Input: part model. Units: mm. Frame: model coordinates. Face numbers are marked on the shaded views. A direction names the side the tool comes from. Coordinates: 2 decimals unless noted, no trailing zeros. Write each loop counter-clockwise with the first axis right and the second up, starting at its lowest first coordinate (ties: lowest second). Pieces come first, ordered by that corner, then holes. Notation, with made-up numbers: M 41,30.25 L 59,30.25 A32 cw 59,60.25 Z; hole C 61.5,-37 d4. An arc over 180 degrees is marked long. Use one line per item in the form item = value.
from build123d import *

# Parameters (mm, degrees)
RECPAT_COUNT       = 2
RECPAT_ANGLE       = 90
BOSS_EXTRU_1_START = 10
ESQUISSE1_R        = 2
BOSS_EXTRU_1_DEPTH = 10


with BuildPart() as part:
    # Fillet1: read off the stored shape, not the designer's step
    # Fillet1 outline → Fillet1 (revolve)
    with BuildSketch(Plane.YX):
        with BuildLine():
            Line((2, 3.3), (2, 8.1))
            Line((2, 8.1), (0, 8.1))
            Line((0, 8.1), (0, 0))
            ThreePointArc((0, 0), (2.027933458, 0.324444488), (3.853420198, 1.265388956))
            ThreePointArc((3.853420198, 1.265388956), (3.961271902, 1.392873227), (4, 1.555305874))
            Line((4, 1.555305874), (4, 3.1))
            Line((4, 3.1), (2.2, 3.1))
            ThreePointArc((2.2, 3.1), (2.058578644, 3.158578644), (2, 3.3))
        make_face()
    revolve(axis=Axis((0, 0, 0), (1, 0, 0)))

    # Sketch3 → Recess section 0
    with BuildSketch(Plane(origin=(0, 0, 0), x_dir=(0, 0, -1), z_dir=(1, 0, 0))):
        with BuildLine():
            Line((0.515, -2.15), (-0.515, -2.15))
            Line((-0.515, -2.15), (-0.515, 2.15))
            Line((-0.515, 2.15), (0.515, 2.15))
            Line((0.515, 2.15), (0.515, -2.15))
        make_face()
    # Sketch4 → Recess section 1
    with BuildSketch(Plane(origin=(2.34, 0, 0), x_dir=(0, 0, -1), z_dir=(1, 0, 0))):
        with BuildLine():
            Line((0.515, -0.983319232), (-0.515, -0.983319232))
            Line((-0.515, -0.983319232), (-0.515, 0.983319232))
            Line((-0.515, 0.983319232), (0.515, 0.983319232))
            Line((0.515, 0.983319232), (0.515, -0.983319232))
        make_face()
    recess = loft(mode=Mode.SUBTRACT)

    # RecPat: Recess ×2 about axis
    recpat_axis = Axis((0, 0, 0), (1, 0, 0))
    for i in range(1, RECPAT_COUNT):
        add(recess.rotate(recpat_axis, i * RECPAT_ANGLE / (RECPAT_COUNT - 1)), mode=Mode.SUBTRACT)

    # RecCorSke → RecessCore (revolve, cut)
    with BuildSketch(Plane.XY, mode=Mode.PRIVATE) as recesscore_sk:
        Polygon((0, 0), (0, 1.01462874), (2.34, 0.851), (2.616506661, 0), align=None)
    revolve(recesscore_sk.sketch.rotate(Axis((-3.175, 0, 0), (1, 0, 0)), 90), axis=Axis((-3.175, 0, 0), (1, 0, 0)), mode=Mode.SUBTRACT)

    # Esquisse1 → Boss.-Extru.1 (add)
    with BuildSketch(Plane(origin=(8.1, 0, 0), x_dir=(0, 0, -1), z_dir=(1, 0, 0)).offset(BOSS_EXTRU_1_START)):
        with Locations(Location((0, 0, 0), (0, 0, 180))):
            Circle(ESQUISSE1_R)
    extrude(amount=-BOSS_EXTRU_1_DEPTH)


solid = part.part
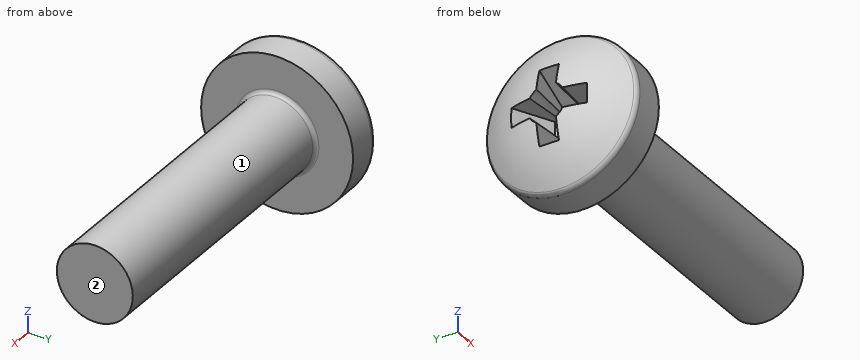
(1) Set-up query: the marked faces 1 and 2. Return all of +Z, -Z, +X, -X, +Y, -Y with unobstructed straight access to the full face (end or side cutting, diameter ignored); none if empty.
Computed:
face_1 = +X
face_2 = +Z, -Z, +X, +Y, -Y
(2) Section query A-A on x = 15. Return the cut outline in (y, z), plus the area to 3 significant figures.
Computed:
outline = C 0,0 d4
area = 12.6 mm^2
(3) First-contact query: pin 1 Ø3 at (x, y) = (3.5, -0.5) entering from -Z; pin 2 Ø1 at (x, y) = (4, -1) entering from +Z; pin 3 Ø4 at (y, z) = (-2.5, -2.5) entering from -X; pin 4 Ø1 at (x, y) = (7.5, 3) entering from +Z. Flat tips, straight axial feed; report the tip coordinate or a pass-through.
Computed:
pin_1 = -4
pin_2 = 1.94
pin_3 = 0.18
pin_4 = through
(4) Line query: probe 1 along Z at (x, y) = (14.25, 0.25); probe 2 along Z at (x, y) = (6.75, 1.75); probe 3 along X at (y, z) = (3, 1). Output: solid intervals per line, ascending.
Computed:
probe_1 = -1.98 to 1.98
probe_2 = -0.97 to 0.97
probe_3 = 0.82 to 3.1
